Geometry: final body of the model. Coordinates: model frame, mm. Round coordinates to 2 decimals unless told otherwise and drop trailing zeros. Loops run counter-clockwise (first coordinate to the right, second up) from the corner with the lowest first, then second, coordinate; pieces in that order, holes last. Notation, with made-up numbers: (20.5, 55.25) -> (52.5, 55.25) arc R23 cw to (52.5, 94.25) -> close; hole circle Ø10 at (-8, 73.5). An arc over 180 degrees is marked (long way). Answer in a Markdown table with one row per item.
```python
from build123d import *

# Parameters (mm, degrees)
F0_R     = 2.15265
F1_DEPTH = 3.175


with BuildPart() as f1:
    # F0 (on Top) → F1 (new body)
    with BuildSketch(Plane.XY):
        with BuildLine():
            ThreePointArc((355.6, 0), (177.8, 177.8), (0, 0))
            Line((0, 0), (0, -139.7))
            ThreePointArc((0, -139.7), (177.8, -317.5), (355.6, -139.7))
            Line((355.6, -139.7), (355.6, 0))
        make_face()
        with Locations((114.497731, -176.317746)):
            Circle(F0_R, mode=Mode.SUBTRACT)
        with Locations((250.03125, -254)):
            Circle(F0_R, mode=Mode.SUBTRACT)
        with Locations((250.03125, -195.2625)):
            Circle(F0_R, mode=Mode.SUBTRACT)
        with Locations((308.76875, -254)):
            Circle(F0_R, mode=Mode.SUBTRACT)
        with Locations((308.76875, -195.2625)):
            Circle(F0_R, mode=Mode.SUBTRACT)
        with Locations((241.102269, -176.317746)):
            Circle(F0_R, mode=Mode.SUBTRACT)
        with Locations((114.497731, 62.017746)):
            Circle(F0_R, mode=Mode.SUBTRACT)
        with Locations((177.8, 96.8375)):
            Circle(F0_R, mode=Mode.SUBTRACT)
        with Locations((241.102269, 62.017746)):
            Circle(F0_R, mode=Mode.SUBTRACT)
        with Locations((177.8, 173.0375)):
            Circle(F0_R, mode=Mode.SUBTRACT)
    extrude(amount=F1_DEPTH)


solid = f1.part
```
Item 1: First-contact query: P1, Ø3, axis at x = 49, y = -169, coming from the -Z side. Flat tip, straight axial feed; report the tip coordinate or a pass-through.
Ans:
| item | result |
|---|---|
| P1 | z = 0 |
Item 2: Section query C-C, the plane y = -268. Output: boundary loops of the cut face in (x, z) (3 decimals), and give its area (3 significant figures).
Ans:
| item | result |
|---|---|
| outline | (54.707, 0) -> (300.893, 0) -> (300.893, 3.175) -> (54.707, 3.175) -> close |
| area | 782 mm2 |
Item 3: Section query A-A, the plane z = 2.5. State how many separate pieces and enclosed holes the cut face has, and give its area (3 significant figures).
Ans:
| item | result |
|---|---|
| separate pieces | 1 |
| enclosed holes | 10 |
| area | 149,000 mm2 |
Item 4: Section query B-B, the plane y = 122. Output: boundary loops of the cut face in (x, z) (3 decimals).
Ans:
| item | result |
|---|---|
| outline | (48.46, 0) -> (307.14, 0) -> (307.14, 3.175) -> (48.46, 3.175) -> close |
Item 5: Ray query, L1, parallel to X at y = 63, z = 0.95; L2, parallel to Y at x = 175.5, z = 0.8; L3, parallel to X at y = 3, z = 0.15. Return the intervals inside material, ascending.
Ans:
| item | result |
|---|---|
| L1 | 11.54 to 112.58, 116.41 to 239.19, 243.02 to 344.06 |
| L2 | -317.49 to 177.79 |
| L3 | 0.03 to 355.57 |
